Here's how the part is built. I have some questions about the finished solid (model axes, mm). A direction names the side the tool comes from. Round coordinates to 2 decimals unless told otherwise and drop trailing zeros. Write each loop counter-clockwise with the first axis right and the second up, starting at its lowest first coordinate (ties: lowest second). Pieces come first, ordered by that corner, then holes. Notation, with made-up numbers: (-32, -17) -> (23, -17) arc R25 cw to (23, 11) -> close; hole circle Ø9 at (31.5, 30.5). An arc over 180 degrees is marked (long way). Answer as CSV lines item,"result".
Autodesk Inventor part; units mm, degrees
ref_plane "YZ Plane" through (0, 0, 0) normal (1, 0, 0) x (0, 1, 0)
ref_plane "XZ Plane" through (0, 0, 0) normal (0, 1, 0) x (-1, 0, 0)
ref_plane "XY Plane" through (0, 0, 0) normal (0, 0, 1) x (1, 0, 0)
sketch "Sketch1" plane through (0, 0, 0) normal (0, 1, 0) x (-1, 0, 0)
  circle A0 centre (0, 0) radius 3
  circle A1 centre (0, 0) radius 4.5
  line L0 (0, 0) -> (7.62, 0) construction
  circle A2 centre (0, 0) radius 1.5
  line L1 (0, 0) -> (0, 4.5) construction
  arc A3 (20.25, -2.4875) -> (20.25, 2.4875) centre (20, 0) ccw
  line L2 (20, 0) -> (0, 0)
  arc A4 (-20.25, 2.4875) -> (-20.25, -2.4875) centre (-20, 0) ccw
  line L3 (20.25, 2.4875) -> (0.45, 4.4774)
  line L4 (20.25, -2.4875) -> (0.45, -4.4774)
  line L5 (-20.25, -2.4875) -> (-0.45, -4.4774)
  line L6 (-20.25, 2.4875) -> (-0.45, 4.4774)
  point P0 (10.62, 0)
  point P1 (13.62, 0)
  point P2 (16.62, 0)
  point P3 (19.62, 0)
  point P4 (-7.62, 0)
  point P5 (-7.62, 0)
  point P6 (-10.62, 0)
  point P7 (-13.62, 0)
  point P8 (-16.62, 0)
  point P9 (-19.62, 0)
  dimension "d0" = 6
  dimension "d1" = 9
  dimension "d2" = 7.62
  dimension "d6" = 3
  dimension "d9" = 3
  dimension "d14" = 2.5
  dimension "d15" = 40
extrude "Extrusion1" add sketch "Sketch1" along normal blind 2 contours A1 | A1 L3 A3 L4 | A1 L5 A4 L6
extrude "Extrusion2" add sketch "Sketch1" against normal blind 1 contours A0 | A1
extrude "Extrusion3" add sketch "Sketch1" against normal blind 4 contours A1
hole "Hole1" at (-7.62, 0, 0) at (-10.62, 0, 0) at (-13.62, 0, 0) at (-16.62, 0, 0) at (-19.62, 0, 0) at (19.62, 0, 0) at (16.62, 0, 0) at (13.62, 0, 0) at (10.62, 0, 0) at (7.62, 0, 0) direction (0, 1, 0) diameter 1.2 depth 8 tip angle 118
sketch "Sketch2" plane through (0, 2, 0) normal (0, 1, 0) x (1, 0, 0)
  circle A0 centre (10.62, 0) radius 0.6
  circle A1 centre (16.62, 0) radius 0.6
  circle A2 centre (19.62, 0) radius 0.6
  circle A3 centre (13.62, 0) radius 0.6
  circle A4 centre (7.62, 0) radius 0.6
  line L0 (0.45, -4.4774) -> (20.25, -2.4875)
  arc A5 (20.25, -2.4875) -> (20.25, 2.4875) centre (20, 0) ccw
  line L1 (20.25, 2.4875) -> (0.45, 4.4774)
  line L2 (7.62, -3.7568) -> (7.62, 3.7568)
extrude "Extrusion4" cut sketch "Sketch2" against normal up to next contours A4 L2 | A4 L2 L1 A5 L0 picked at (7.7764, 0.1247)
properties part number "servo arm HK15138 2 cut to 1"
1. On a 3-axis mill with a long thin cutter (end or side, diameter ignored), from which of +Z, -Z, +X, -X, +Y, -Y can I reach the whole of each face in a straight line? I mean faces 5 (the face through (6, 0, 0)), 6 (the face through (3, 1, 0)), 7 (the face through (4.09, 0.99, 4.11)), 8 (the face through (-1.3, -1, -1.3)), 9 (the face through (-19.1, 1, -0.3)). Say none if no direction works.
Numbers:
face 5,"+X, -Y"
face 6,"+Y"
face 7,"+Z, +X, +Y, -Y"
face 8,"-Y"
face 9,"+Y, -Y"
2. Suppose I cut it at D-D on y = -3.2. Please give me the cut outline in (x, z), and give its area (3 significant figures).
Numbers:
outline,"circle Ø9 at (0, 0); hole circle Ø6 at (0, 0)"
area,"35.3 mm^2"
3. Suppose I cut it at B-B on y = 0.6. Please give me the cut outline in (x, z).
Numbers:
outline,"(-20.25, -2.49) -> (-0.45, -4.48) arc R4.5 ccw to (0.45, -4.48) -> (7.62, -3.76) -> (7.62, -0.6) arc R0.6 cw to (7.62, 0.6) -> (7.62, 3.76) -> (0.45, 4.48) arc R4.5 ccw to (-0.45, 4.48) -> (-20.25, 2.49) arc R2.5 ccw to start; hole circle Ø1.2 at (-19.62, 0); hole circle Ø1.2 at (-16.62, 0); hole circle Ø1.2 at (-13.62, 0); hole circle Ø1.2 at (-10.62, 0); hole circle Ø1.2 at (-7.62, 0); hole circle Ø6 at (0, 0)"
4. Suppose I cut it at A-A on x = 0. Please give me the cut outline in (y, z).
Numbers:
outline,"(-4, -4.5) -> (2, -4.5) -> (2, -3) -> (0, -3) -> (0, -1.5) -> (-1, -1.5) -> (-1, -3) -> (-4, -3) -> close; (-4, 3) -> (-1, 3) -> (-1, 1.5) -> (0, 1.5) -> (0, 3) -> (2, 3) -> (2, 4.5) -> (-4, 4.5) -> close"
5. If I drill on line 1 (Z direction, x = 0, y = -3.1); line 2 (Z direction, x = 0, y = -0.4); line 3 (X direction, y = -0.4, z = 3.75), over which ranges is the centre line in solid material (lowest first)?
Numbers:
line 1,"z = -4.5 to -3, 3 to 4.5"
line 2,"z = -4.5 to -1.5, 1.5 to 4.5"
line 3,"x = -2.49 to 2.49"
6. Suppose I cut it at C-C on x = -13.62. Please give me the cut outline in (y, z).
Numbers:
outline,"(0, -3.15) -> (2, -3.15) -> (2, -0.6) -> (0, -0.6) -> close; (0, 0.6) -> (2, 0.6) -> (2, 3.15) -> (0, 3.15) -> close"
7. For pin 1 Ø1 at (y, z) = (1, -2) entering from -X; pin 2 Ø1.6 at (x, z) = (-7.62, 0) entering from -Y; pin 3 Ø3 at (x, y) = (3.5, 0) entering from +Z; pin 4 Ø5 at (x, z) = (-1, 0.5) entering from +Y, each with a flat end and sliding along its axis, tell me the tip position at first contact or that it passes through.
Numbers:
pin 1,"stops at x = -22"
pin 2,"stops at y = 0"
pin 3,"stops at z = 4.32"
pin 4,"stops at y = 2"
8. If we mould it in two halves opening along X, with no side actions, what happens to faces 1 (the face through (3, -2, 0)), 2 (the face through (-22.5, 1, 0.1)), 3 (the face through (-1, -4, -3)), 4 (the face through (0.59, -1.62, 4.46))? For each: released by +X, released by -X, zero draft, split by the parting line, or undercut.
Numbers:
face 1,"undercut"
face 2,"released by -X"
face 3,"zero draft"
face 4,"split by the parting line"
